Autodesk Inventor part; units mm, degrees
ref_plane "YZ Plane" through (0, 0, 0) normal (1, 0, 0) x (0, 1, 0)
ref_plane "XZ Plane" through (0, 0, 0) normal (0, 1, 0) x (-1, 0, 0)
ref_plane "XY Plane" through (0, 0, 0) normal (0, 0, 1) x (1, 0, 0)
sketch "Sketch1" plane through (0, 0, 0) normal (0, 0, 1) x (1, 0, 0)
  arc A0 (330.1893, 100) -> (-323.606, 119.6) centre (0, 0) ccw
  line L0 (-351.7456, 100) -> (-921.7456, 100)
  arc A1 (-351.7456, 100) -> (-323.606, 119.6) centre (-351.7456, 130) ccw
  arc A2 (340.6244, 100) -> (-332.9859, 123.0667) centre (0, 0) ccw
  line L1 (-921.7456, 100) -> (-921.7456, 110)
  line L2 (-921.7456, 110) -> (-351.7456, 110)
  arc A3 (-351.7456, 110) -> (-332.9859, 123.0667) centre (-351.7456, 130) ccw
  line L3 (0, 0) -> (0, 130)
  line L4 (330.1893, 100) -> (340.6244, 100)
  point P0 (330.3407, 130)
  dimension "d25" = 130
  dimension "d26" = 20
  dimension "d27" = 30
  dimension "d28" = 570
  dimension "d29" = 345
  dimension "d30" = 100
extrude "Extrusion1" add sketch "Sketch1" along normal blind 175
properties part number "carril1"
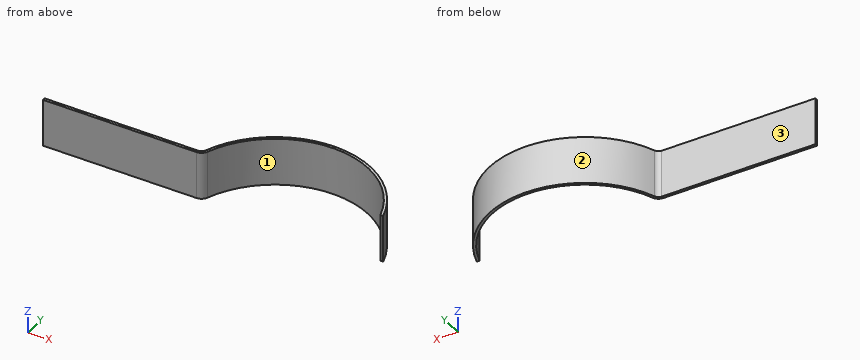
Design review of the part built by this model. Coordinates are the model's own, in mm. Face numbers are marked on the shaded views. Round coordinates to 2 decimals unless told otherwise and drop trailing zeros. Write each loop counter-clockwise with the first axis right and the second up, starting at its lowest first coordinate (ties: lowest second). Pieces come first, ordered by that corner, then holes.
Item 1: Consider section D-D on y = 153.5. Give the boundary of the cut face in (x, z), and give its area (3 significant figures).
Item 2: Consider section C-C on x = -492. Give the boundary of the cut face in (y, z), and give its area (3 significant figures).
Item 3: Consider section B-B on z = 161. Give the boundary of the cut face in (x, y), and give its area (3 significant figures).
Item 4: Draft analysis for pull direction X (two halves, no side actions). For the marked faces 1, 2 and 3, state which applies: released by +X, released by -X, zero draft, split by the parting line, or undercut.
Item 5: Wall thickness on L1, parallel to Y at x = -632.5, z = 32.5; L2, parallel to X at y = 319, z = 56.5; L3, parallel to X at y = 225, z = 59.5: over which ranges is each line inside the solid? List them lowest first.
Item 6: For pin 1 Ø3 at (x, z) = (-256.5, 45) entering from +Y; pin 2 Ø5 at (y, z) = (276.5, 70.5) entering from -X; pin 3 Ø1.5 at (y, z) = (296.5, 18.5) entering from -X, all flat-tipped, find the tip position at first contact; note any pin that passes through.
Item 7: Consider section A-A on y = 302. Give the boundary of the cut face in (x, z).
Check values:
1. outline: (-320.1, 0) - (-308.97, 0) - (-308.97, 175) - (-320.1, 175) - close; (308.97, 0) - (320.1, 0) - (320.1, 175) - (308.97, 175) - close
1. area: 3,890 mm2
2. outline: (100, 0) - (110, 0) - (110, 175) - (100, 175) - close
2. area: 1,750 mm2
3. outline: (-921.75, 100) - (-351.75, 100) arc R30 ccw to (-323.61, 119.6) arc R345 cw to (330.19, 100) - (340.62, 100) arc R355 ccw to (-332.99, 123.07) arc R20 cw to (-351.75, 110) - (-921.75, 110) - close
3. area: 14,700 mm2
4. face 1: undercut
4. face 2: split by the parting line
4. face 3: zero draft
5. L1: y = 100 to 110
5. L2: x = -155.77 to -131.39, 131.39 to 155.77
5. L3: x = -274.59 to -261.53, 261.53 to 274.59
6. pin 1: stops at y = 246.98
6. pin 2: stops at x = -225.72
6. pin 3: stops at x = -196.36
7. outline: (-186.6, 0) - (-166.8, 0) - (-166.8, 175) - (-186.6, 175) - close; (166.8, 0) - (186.6, 0) - (186.6, 175) - (166.8, 175) - close
